Could you check a few things on this drawing? It's one solid part, dimensions in mm from its lowest x, y, z. Coordinates: 2 decimals unless noted, no trailing zeros. Write each loop counter-clockwise with the first axis right and the second up, starting at its lowest first coordinate (ties: lowest second). Pieces come first, ordered by that corner, then holes. Notation, with made-up numbers: (42, 39.25) - (57, 39.25) arc R24 ccw to (57, 75.25) - close; hole circle Ø2 at (48.5, 70). An arc over 180 degrees is marked (long way). Answer as a JSON object with one key per item and string values. Group by question number.
1) Please list where these lines run through material, in increasing order: line 1 along Y through (x, z) = (12.5, 1.25); line 2 along Y through (x, z) = (2.75, 2.5); line 3 along X through (y, z) = (0.95, 15).
2) Will this pin go through, and if not, where does the flat tip stop? pin 1 Ø5 at (x, y) = (19.5, 22.25) entering from +Z.
3) If we section it at A-A (z = 10.75): Write out the boundary of the cut face in (x, y).
4) If we section it at C-C (x = 5.5): Write out the boundary of the cut face in (y, z), plus the area to 3 significant figures.
5) If we section it at B-B (x = 12.5): Write out the boundary of the cut face in (y, z).
6) We'd pull the mould along Y, two halves only. Please class the marked faces 1, 2, 3 and 4: released by +Y, released by -Y, zero draft, split by the parting line, or undercut.
7) If we section it at D-D (y = 22.25): Write out the boundary of the cut face in (x, z), plus the area to 3 significant figures.
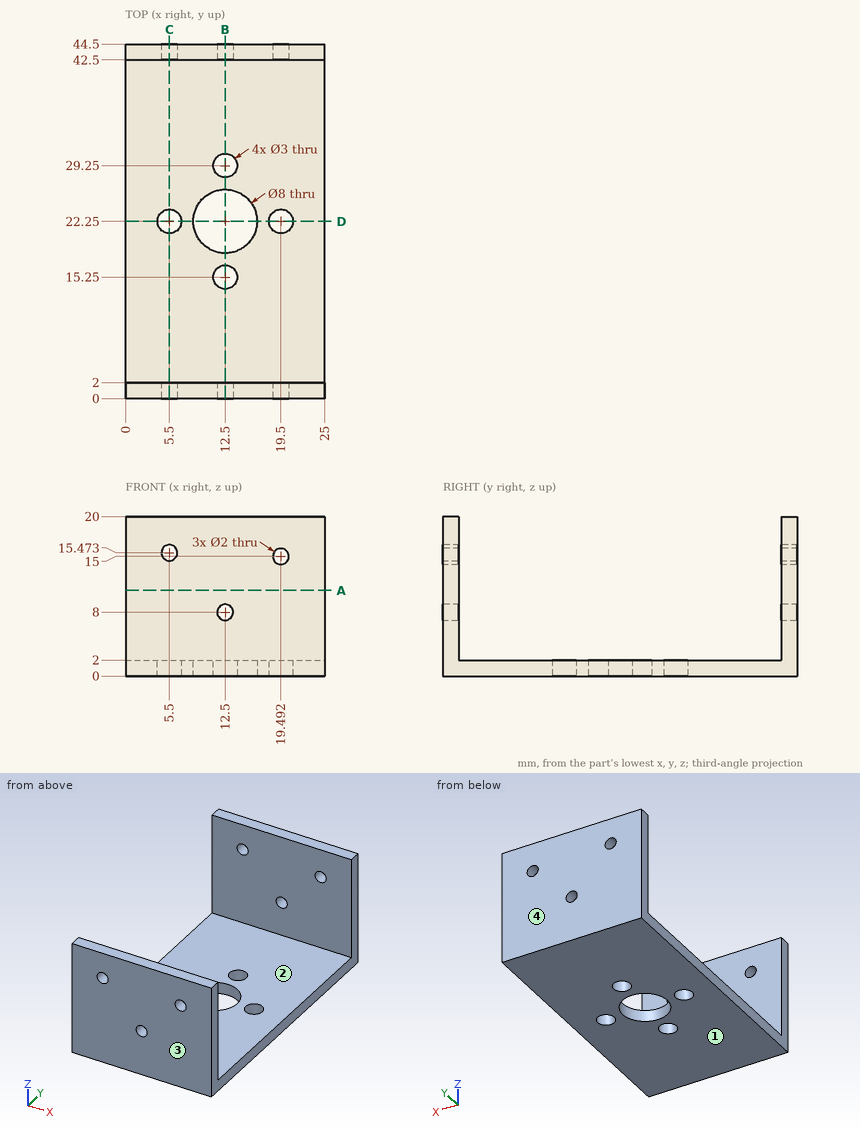
Here are the results:
{
 "1": {"line 1": "y = 0 to 13.75, 16.75 to 18.25, 26.25 to 27.75, 30.75 to 44.5", "line 2": "y = 0 to 2, 42.5 to 44.5", "line 3": "x = 0 to 4.62, 6.38 to 18.49, 20.49 to 25"},
 "2": {"pin 1": "stops at z = 2"},
 "3": {"outline": "(0, 0) - (25, 0) - (25, 2) - (0, 2) - close; (0, 42.5) - (25, 42.5) - (25, 44.5) - (0, 44.5) - close"},
 "4": {"outline": "(0, 0) - (20.75, 0) - (20.75, 2) - (2, 2) - (2, 14.47) - (0, 14.47) - close; (0, 16.47) - (2, 16.47) - (2, 20) - (0, 20) - close; (23.75, 0) - (44.5, 0) - (44.5, 14.47) - (42.5, 14.47) - (42.5, 2) - (23.75, 2) - close; (42.5, 16.47) - (44.5, 16.47) - (44.5, 20) - (42.5, 20) - close", "area": "147 mm²"},
 "5": {"outline": "(0, 0) - (13.75, 0) - (13.75, 2) - (2, 2) - (2, 7) - (0, 7) - close; (0, 9) - (2, 9) - (2, 20) - (0, 20) - close; (16.75, 0) - (18.25, 0) - (18.25, 2) - (16.75, 2) - close; (26.25, 0) - (27.75, 0) - (27.75, 2) - (26.25, 2) - close; (30.75, 0) - (44.5, 0) - (44.5, 7) - (42.5, 7) - (42.5, 2) - (30.75, 2) - close; (42.5, 9) - (44.5, 9) - (44.5, 20) - (42.5, 20) - close"},
 "6": {"face 1": "zero draft", "face 2": "undercut", "face 3": "released by -Y", "face 4": "released by +Y"},
 "7": {"outline": "(0, 0) - (4, 0) - (4, 2) - (0, 2) - close; (7, 0) - (8.5, 0) - (8.5, 2) - (7, 2) - close; (16.5, 0) - (18, 0) - (18, 2) - (16.5, 2) - close; (21, 0) - (25, 0) - (25, 2) - (21, 2) - close", "area": "22.0 mm²"}
}
